```python
from build123d import *

# Parameters (mm, degrees)
SKETCH_W     = 120
SKETCH_H     = 80
SKETCH_R     = 2.5
PAD_DEPTH    = 1.8
SKETCH001_R  = 2.5
PAD001_DEPTH = 4


with BuildPart() as part:
    # Sketch → Pad (new body)
    with BuildSketch(Plane.XY):
        with Locations((60, 40)):
            Rectangle(SKETCH_W, SKETCH_H)
        with Locations((8.5, 4.5)):
            Circle(SKETCH_R, mode=Mode.SUBTRACT)
        with Locations((48.5, 4.5)):
            Circle(SKETCH_R, mode=Mode.SUBTRACT)
        with Locations((88.5, 4.5)):
            Circle(SKETCH_R, mode=Mode.SUBTRACT)
        with Locations((28.5, 14.5)):
            Circle(SKETCH_R, mode=Mode.SUBTRACT)
        with Locations((108.5, 14.5)):
            Circle(SKETCH_R, mode=Mode.SUBTRACT)
        with Locations((8.5, 24.5)):
            Circle(SKETCH_R, mode=Mode.SUBTRACT)
        with Locations((48.5, 24.5)):
            Circle(SKETCH_R, mode=Mode.SUBTRACT)
        with Locations((88.5, 24.5)):
            Circle(SKETCH_R, mode=Mode.SUBTRACT)
        with Locations((8.5, 44.5)):
            Circle(SKETCH_R, mode=Mode.SUBTRACT)
        with Locations((48.5, 44.5)):
            Circle(SKETCH_R, mode=Mode.SUBTRACT)
        with Locations((88.5, 44.5)):
            Circle(SKETCH_R, mode=Mode.SUBTRACT)
        with Locations((28.5, 54.5)):
            Circle(SKETCH_R, mode=Mode.SUBTRACT)
        with Locations((68.5, 54.5)):
            Circle(SKETCH_R, mode=Mode.SUBTRACT)
        with Locations((108.5, 54.5)):
            Circle(SKETCH_R, mode=Mode.SUBTRACT)
        with Locations((88.5, 64.5)):
            Circle(SKETCH_R, mode=Mode.SUBTRACT)
        with Locations((48.5, 64.5)):
            Circle(SKETCH_R, mode=Mode.SUBTRACT)
        with Locations((8.5, 64.5)):
            Circle(SKETCH_R, mode=Mode.SUBTRACT)
        with Locations((28.5, 34.5)):
            Circle(SKETCH_R, mode=Mode.SUBTRACT)
        with Locations((68.5, 34.5)):
            Circle(SKETCH_R, mode=Mode.SUBTRACT)
        with Locations((108.5, 34.5)):
            Circle(SKETCH_R, mode=Mode.SUBTRACT)
        with Locations((28.5, 74.5)):
            Circle(SKETCH_R, mode=Mode.SUBTRACT)
        with Locations((68.5, 74.5)):
            Circle(SKETCH_R, mode=Mode.SUBTRACT)
        with Locations((108.5, 74.5)):
            Circle(SKETCH_R, mode=Mode.SUBTRACT)
        with Locations((68.5, 14.5)):
            Circle(SKETCH_R, mode=Mode.SUBTRACT)
    extrude(amount=PAD_DEPTH)

    # Sketch001 (on Face30 of Pad) → Pad001 (join)
    with BuildSketch(Plane.XY.offset(1.8)):
        Polygon((0.060355, 74.846256), (0.060355, 24.889119), (5.060355, 19.889119), (26.945464, 19.889119), (32.518221, 25.461876), (32.518221, 39.837159), (38.816962, 46.1359), (92.724373, 46.1359), (97.724373, 51.1359), (97.724373, 75), (92.724373, 80), (69, 80), (53.943623, 95.103615), (30.079678, 95.103615), (14.912183, 79.846256), (5.060355, 79.846256), align=None)
        with Locations((8.485094, 64.523872)):
            Circle(SKETCH001_R, mode=Mode.SUBTRACT)
        with Locations((28.521502, 34.481613)):
            Circle(SKETCH001_R, mode=Mode.SUBTRACT)
        with Locations((88.466942, 64.525024)):
            Circle(SKETCH001_R, mode=Mode.SUBTRACT)
    extrude(amount=PAD001_DEPTH)


solid = part.part
```
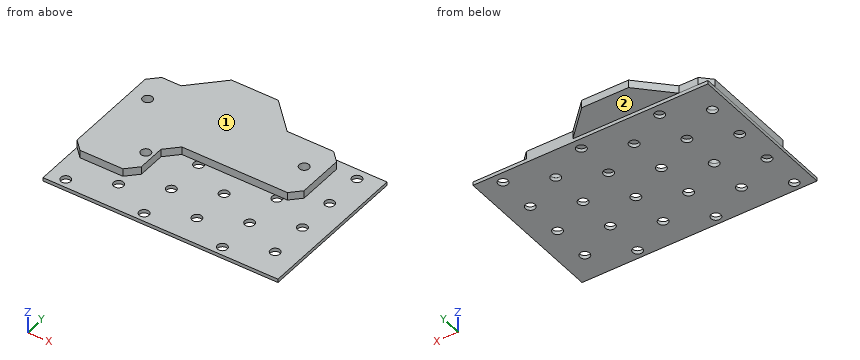
Geometry: final body of the model. Coordinates: model frame, mm. Face numbers are marked on the shaded views. A direction names the side the tool comes from. Round coordinates to 2 decimals unless told otherwise and drop trailing zeros. Write each loop counter-clockwise with the first axis right and the second up, starting at its lowest first coordinate (ties: lowest second). Pieces come first, ordered by that corner, then holes. Notation, with made-up numbers: (1.5, 34) -> (24.5, 34) arc R29 ccw to (24.5, 62) -> close; hole circle Ø1 at (62.5, 30.25). An arc over 180 degrees is marked (long way). Return JSON: item names as keys, results as strings.
Q1. First-contact query: pin 1 Ø5.5 at (x, y) = (7.5, 23.5) entering from -Z; pin 2 Ø8 at (x, y) = (48.5, 4.5) entering from +Z; pin 3 Ø2 at (x, z) = (42, 3) entering from -Y; pin 4 Ø2 at (x, z) = (12, 3.5) entering from +Y. Flat tips, straight axial feed; report the tip coordinate or a pass-through.
From the geometry:
{"pin 1": "z = 0", "pin 2": "z = 1.8", "pin 3": "y = 46.14", "pin 4": "y = 79.85"}
Q2. Section D-D on z = 3.9. Return the cut outline in (x, y).
From the geometry:
{"outline": "(0.06, 24.89) -> (5.06, 19.89) -> (26.95, 19.89) -> (32.52, 25.46) -> (32.52, 39.84) -> (38.82, 46.14) -> (92.72, 46.14) -> (97.72, 51.14) -> (97.72, 75) -> (92.72, 80) -> (69, 80) -> (53.94, 95.1) -> (30.08, 95.1) -> (14.91, 79.85) -> (5.06, 79.85) -> (0.06, 74.85) -> close; hole circle Ø5 at (8.49, 64.52); hole circle Ø5 at (28.52, 34.48); hole circle Ø5 at (88.47, 64.53)"}
Q3. Section B-B on y = 54.5. Return the cut outline in (x, z), and give its area (3 significant figures).
From the geometry:
{"outline": "(0, 0) -> (26, 0) -> (26, 1.8) -> (31, 1.8) -> (31, 0) -> (66, 0) -> (66, 1.8) -> (71, 1.8) -> (71, 0) -> (106, 0) -> (106, 1.8) -> (97.72, 1.8) -> (97.72, 5.8) -> (0.06, 5.8) -> (0.06, 1.8) -> (0, 1.8) -> close; (111, 0) -> (120, 0) -> (120, 1.8) -> (111, 1.8) -> close", "area": "580 mm2"}
Q4. Section A-A on x = 108.5. Return the cut outline in (y, z), and give its area (3 significant figures).
From the geometry:
{"outline": "(0, 0) -> (12, 0) -> (12, 1.8) -> (0, 1.8) -> close; (17, 0) -> (32, 0) -> (32, 1.8) -> (17, 1.8) -> close; (37, 0) -> (52, 0) -> (52, 1.8) -> (37, 1.8) -> close; (57, 0) -> (72, 0) -> (72, 1.8) -> (57, 1.8) -> close; (77, 0) -> (80, 0) -> (80, 1.8) -> (77, 1.8) -> close", "area": "108 mm2"}
Q5. Ray query, line 1 (Y direction, x = 68.5, z = 0.95); line 2 (Y direction, x = 8.5, z = 0.4); line 3 (Z direction, x = 82, y = 27.5). Return the intervals inside material, ascending.
From the geometry:
{"line 1": "0 to 12, 17 to 32, 37 to 52, 57 to 72, 77 to 80", "line 2": "0 to 2, 7 to 22, 27 to 42, 47 to 62, 67 to 80", "line 3": "0 to 1.8"}
Q6. Section C-C on x = 28.5. Give the number of separate pieces and of enclosed holes in the cut face, and give its area (3 significant figures).
From the geometry:
{"separate pieces": "3", "enclosed holes": "0", "area": "376 mm2"}
Q7. Set-up query: the marked faces 1 and 2. Return all of +Z, -Z, +X, -X, +Y, -Y with unobstructed straight access to the full face (end or side cutting, diameter ignored); none if empty.
From the geometry:
{"face 1": "+Z, +X, -X, +Y, -Y", "face 2": "-Z, +X, -X, +Y"}
